Autodesk Inventor part; units mm, degrees
ref_plane "YZ Plane" through (0, 0, 0) normal (1, 0, 0) x (0, 1, 0)
ref_plane "XZ Plane" through (0, 0, 0) normal (0, 1, 0) x (-1, 0, 0)
ref_plane "XY Plane" through (0, 0, 0) normal (0, 0, 1) x (1, 0, 0)
sketch "Sketch1" plane through (0, 0, 0) normal (0, 1, 0) x (-1, 0, 0)
  line L0 (0, 0) -> (-54, 0)
  line L1 (-54, 0) -> (-54, -77)
  line L2 (-54, -77) -> (0, -77)
  line L3 (0, -77) -> (0, 0)
  dimension "d0" = 77
  dimension "d1" = 54
extrude "Extrusion1" add sketch "Sketch1" along normal blind 4.5
sketch "Sketch2" plane through (0, 4.5, 0) normal (0, 1, 0) x (1, 0, 0)
  line L0 (4.5, 4.5) -> (49.5, 4.5) construction
  line L1 (49.5, 4.5) -> (49.5, 72.5) construction
  line L2 (49.5, 72.5) -> (4.5, 72.5) construction
  line L3 (4.5, 72.5) -> (4.5, 4.5) construction
  circle A0 centre (4.5, 4.5) radius 2
  circle A1 centre (17.5, 4.5) radius 2
  circle A2 centre (36.5, 4.5) radius 2
  circle A3 centre (49.5, 4.5) radius 2
  circle A4 centre (4.5, 17.5) radius 2
  circle A5 centre (4.5, 31.5) radius 2
  circle A6 centre (4.5, 59.5) radius 2
  circle A7 centre (4.5, 72.5) radius 2
  circle A8 centre (17.5, 72.5) radius 2
  circle A9 centre (36.5, 72.5) radius 2
  circle A10 centre (49.5, 72.5) radius 2
  circle A11 centre (49.5, 59.5) radius 2
  circle A12 centre (49.5, 45.5) radius 2
  circle A13 centre (49.5, 31.5) radius 2
  circle A14 centre (49.5, 17.5) radius 2
  line L4 (54, 0) -> (54, 77)
  line L5 (0, 0) -> (54, 0)
  line L6 (54, 77) -> (0, 77)
  line L7 (0, 77) -> (0, 0)
  circle A15 centre (4.5, 45.5) radius 2
  dimension "d4" = 4
  dimension "d5" = 4
  dimension "d6" = 4
  dimension "d7" = 4
  dimension "d8" = 4
  dimension "d9" = 4
  dimension "d11" = 4
  dimension "d12" = 4
  dimension "d13" = 4
  dimension "d14" = 4
  dimension "d15" = 4
  dimension "d16" = 4
  dimension "d17" = 4
  dimension "d18" = 4
  dimension "d19" = 4
  dimension "d20" = 4.5
  dimension "d21" = 4.5
  dimension "d22" = 4.5
  dimension "d23" = 4.5
  dimension "d24" = 13
  dimension "d25" = 14
  dimension "d26" = 13
  dimension "d27" = 4
  dimension "d28" = 14
  dimension "d29" = 13
  dimension "d30" = 19
  dimension "d31" = 13
  dimension "d32" = 14
  dimension "d33" = 14
  dimension "d34" = 14
  dimension "d35" = 13
  dimension "d36" = 19
hole "Hole1" at (4.5, 4.5, -4.5) at (17.5, 4.5, -4.5) at (4.5, 4.5, -17.5) at (36.5, 4.5, -4.5) at (4.5, 4.5, -31.5) at (49.5, 4.5, -4.5) at (49.5, 4.5, -17.5) at (4.5, 4.5, -45.5) at (4.5, 4.5, -59.5) at (4.5, 4.5, -72.5) at (17.5, 4.5, -72.5) at (36.5, 4.5, -72.5) at (49.5, 4.5, -72.5) at (49.5, 4.5, -59.5) at (49.5, 4.5, -45.5) at (49.5, 4.5, -31.5) direction (0, -1, 0) diameter 4 depth 10 tip angle 118
properties part number "1-35" material "Bronze, Soft Tin"
Can you work these out from the model? Positions are in its coordinate system, mm. Give positions to 0.01 mm unless a question says otherwise; leave off trailing zeros. Loops run counter-clockwise (first coordinate to the right, second up) from the corner with the lowest first, then second, coordinate; pieces in that order, holes last. Notation, with made-up numbers: M 87,46 L 101,46 A13 ccw 101,63 Z; hole C -34.5,6.5 d8. An arc over 180 degrees is marked long. One line per question, with ' | ' between items. Start each with the question number.
Q1. If I drill on line 1 (X direction, y = 3.45, z = -72.5); line 2 (Z direction, x = 17.5, y = 2.7); line 3 (X direction, y = 1.55, z = -17.5), over which ranges is the centre line in solid material (lowest first)? Write a range as from..to.
Q2. If we section it at D-D (x = 49.5): Please give me the cut outline in (y, z).
Q3. If we section it at A-A (z = -31.5): Please give me the cut outline in (x, y).
Q4. If we section it at B-B (y = 2.45): State how many separate pieces and enclosed holes the cut face has, plus the area to 3 significant figures.
Q5. If we mould it in two halves opening along Z, with no side actions, what happens to faces 1 (the flat face through (27, 2, 0)), 2 (the flat face through (0, 2, -39)), 3 (the cylindrical face through (51.452, 2.218, -4.934))? For each: +Z half, -Z half, draft (parallel to the pull), parting line (faces both ways), or undercut.
Q6. If we section it at C-C (x = 36.5): Please give me the cut outline in (y, z), plus the area to 4 significant figures.
Q7. For pin 1 Ø2.5 at (x, z) = (49.5, -4.5) entering from +Y, with a flat end and sliding along its axis, tell me the tip position at first contact or that it passes through.
Computed:
1) line 1: x = 0..2.5, 6.5..15.5, 19.5..34.5, 38.5..47.5, 51.5..54 | line 2: z = -77..-74.5, -70.5..-6.5, -2.5..0 | line 3: x = 0..2.5, 6.5..47.5, 51.5..54
2) outline: M 0,-77 L 4.5,-77 L 4.5,-74.5 L 0,-74.5 Z; M 0,-70.5 L 4.5,-70.5 L 4.5,-61.5 L 0,-61.5 Z; M 0,-57.5 L 4.5,-57.5 L 4.5,-47.5 L 0,-47.5 Z; M 0,-43.5 L 4.5,-43.5 L 4.5,-33.5 L 0,-33.5 Z; M 0,-29.5 L 4.5,-29.5 L 4.5,-19.5 L 0,-19.5 Z; M 0,-15.5 L 4.5,-15.5 L 4.5,-6.5 L 0,-6.5 Z; M 0,-2.5 L 4.5,-2.5 L 4.5,0 L 0,0 Z
3) outline: M 0,0 L 2.5,0 L 2.5,4.5 L 0,4.5 Z; M 6.5,0 L 47.5,0 L 47.5,4.5 L 6.5,4.5 Z; M 51.5,0 L 54,0 L 54,4.5 L 51.5,4.5 Z
4) separate pieces: 1 | enclosed holes: 16 | area: 3,960 mm²
5) face 1: +Z half | face 2: draft | face 3: undercut
6) outline: M 0,-77 L 4.5,-77 L 4.5,-74.5 L 0,-74.5 Z; M 0,-70.5 L 4.5,-70.5 L 4.5,-6.5 L 0,-6.5 Z; M 0,-2.5 L 4.5,-2.5 L 4.5,0 L 0,0 Z | area: 310.5 mm²
7) pin 1: passes through
